from build123d import *

# Parameters (mm, degrees)
F0_R          = 12.7
F0_R_2        = 9.525
F1_DEPTH      = 38.1
F1_DEPTH_BACK = 38.1
F2_SIZE       = 1.016
F3_SIZE       = 0.508


with BuildPart() as f1:
    # F0 (on Front) → F1 (new body, two sides)
    with BuildSketch(Plane.XZ) as f1_sk:
        Circle(F0_R)
        Circle(F0_R_2, mode=Mode.SUBTRACT)
    extrude(amount=F1_DEPTH)
    extrude(f1_sk.sketch, amount=-F1_DEPTH_BACK)

    # F2
    f2_edges = [f1.edges().sort_by_distance(p)[0] for p in [
        (-9.525, -38.1, 0),
        (-9.525, 38.1, 0),
    ]]
    chamfer(f2_edges, length=F2_SIZE)

    # F3
    f3_edges = [f1.edges().sort_by_distance(p)[0] for p in [
        (-12.7, 38.1, 0),
        (-12.7, -38.1, 0),
    ]]
    chamfer(f3_edges, length=F3_SIZE)


solid = f1.part
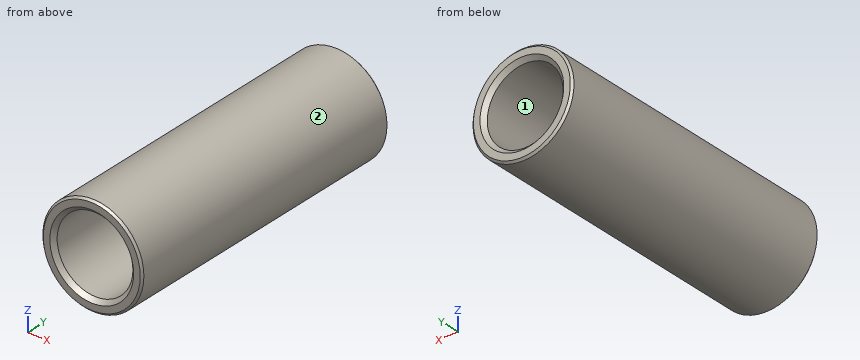
Work out the finished part from the listing and answer in its coordinate system (mm). Face numbers are marked on the shaded views. Give positions to 0.01 mm unless a question says otherwise; leave off trailing zeros. Order: outer loops, then holes, each group sorted by start corner. A loop starts at its lowest first (then second) coordinate and runs counter-clockwise, first axis right, second up. Notation, with made-up numbers: (-15, 28) -> (40, 28) arc R33 ccw to (40, 56) -> close; hole circle Ø2 at (-21, 38.25). An arc over 180 degrees is marked (long way). One line per item, written item: value.
Item 1: Determine the mould class of the marked faces 1 and 2 for opening direction X: released by +X, released by -X, zero draft, split by the parting line, or undercut.
Answer sheet:
face 1: undercut
face 2: split by the parting line
Item 2: Find section C-C, the plane y = 24. Give the vertices of the cut face in (x, z) (3 decimals).
Answer sheet:
outline: circle Ø25.4 at (0, 0); hole circle Ø19.05 at (0, 0)
Item 3: Find section A-A, the plane x = 0. Give the vertices of the cut face in (y, z) (3 decimals), plus the area to 3 significant figures.
Answer sheet:
outline: (-38.1, -12.192) -> (-37.592, -12.7) -> (37.592, -12.7) -> (38.1, -12.192) -> (38.1, -10.541) -> (37.084, -9.525) -> (-37.084, -9.525) -> (-38.1, -10.541) -> close; (-38.1, 10.541) -> (-37.084, 9.525) -> (37.084, 9.525) -> (38.1, 10.541) -> (38.1, 12.192) -> (37.592, 12.7) -> (-37.592, 12.7) -> (-38.1, 12.192) -> close
area: 481 mm²
Item 4: Find section B-B, the plane z = 0. Give the vertices of the cut face in (x, y) (3 decimals).
Answer sheet:
outline: (-12.7, -37.592) -> (-12.192, -38.1) -> (-10.541, -38.1) -> (-9.525, -37.084) -> (-9.525, 37.084) -> (-10.541, 38.1) -> (-12.192, 38.1) -> (-12.7, 37.592) -> close; (9.525, -37.084) -> (10.541, -38.1) -> (12.192, -38.1) -> (12.7, -37.592) -> (12.7, 37.592) -> (12.192, 38.1) -> (10.541, 38.1) -> (9.525, 37.084) -> close
Item 5: Flat-ended cylindrical pins translate along their axes: P1, Ø2, axis at x = -5, y = -28, coming from the +Z side; P2, Ø4, axis at x = 6, z = -2, coming from the -Y side; P3, Ø8, axis at y = 16.5, z = 8.5, coming from the -X side. Find the tip coordinate at first contact, or state that the pin passes through.
Answer sheet:
P1: z = 12.05
P2: through
P3: x = -11.88
Item 6: Straight lines are drawn through the part: probe 1 along X at (y, z) = (14.5, -0.25); probe 2 along Z at (x, y) = (0, 15.5) (3 decimals); probe 3 along X at (y, z) = (1, 5). For each, find the intervals that lie inside material, in ascending order.
Answer sheet:
probe 1: -12.7 to -9.52, 9.52 to 12.7
probe 2: -12.7 to -9.525, 9.525 to 12.7
probe 3: -11.67 to -8.11, 8.11 to 11.67
